The listing builds one solid part. Answer for the finished solid, in the listing's coordinates (mm). A direction names the side the tool comes from. Coordinates: 2 decimals unless noted, no trailing zeros. Order: outer loops, then holes, each group sorted by start corner. A loop starts at its lowest first (then second) coordinate and runs counter-clockwise, first axis right, second up. Notation, with made-up numbers: (-34, 6) -> (3, 6) arc R20 cw to (3, 21) -> close; hole circle Ø3 at (68.25, -1). An arc over 180 degrees is marked (long way). Write item = value, one per line.
from build123d import *

# Parameters (mm, degrees)
F0_W      = 96
F0_H      = 90
F1_DEPTH  = 18
F2_W      = 72
F2_H      = 38
F4_DEPTH  = 67
F6_DEPTH  = 38
F7_W      = 8
F7_H      = 12
F8_DEPTH  = 51.001
F10_DEPTH = 72.001
F11_W     = 20
F11_H     = 5
F12_DEPTH = 96
F13_W     = 46
F13_H     = 26
F14_DEPTH = 5
F16_DEPTH = 3
F17_W     = 3
F17_H     = 14
F18_DEPTH = 72
F19_R     = 2.99999


# Not quite as in the source:
# - a fillet or chamfer is up to 0.001 mm smaller than in the source, because OpenCascade refuses the exact size


with BuildPart() as f1:
    # F0 (on Top) → F1 (new body)
    with BuildSketch(Plane.XY):
        with Locations((48, 45)):
            Rectangle(F0_W, F0_H)
    extrude(amount=F1_DEPTH)

    # F2 (on face) → F4 (join, through all)
    with BuildSketch(Plane.XY.offset(18)):
        with Locations((48, 71)):
            Rectangle(F2_W, F2_H)
    extrude(amount=F4_DEPTH)

    # F5 (on face) → F6 (cut, through all)
    with BuildSketch(Plane.XZ.offset(-52)):
        Polygon((84, 52), (84, 85), (51, 85), align=None)
    extrude(amount=-F6_DEPTH, mode=Mode.SUBTRACT)

    # F7 (on face) → F8 (cut, through all)
    with BuildSketch(Plane(origin=(12, 0, 0), x_dir=(0, -1, 0), z_dir=(-1, 0, 0))):
        with Locations((-64, 79)):
            Rectangle(F7_W, F7_H)
    extrude(amount=-F8_DEPTH, mode=Mode.SUBTRACT)

    # F9 (on face) → F10 (cut, through all)
    with BuildSketch(Plane(origin=(12, 0, 0), x_dir=(0, -1, 0), z_dir=(-1, 0, 0))):
        Polygon((-90, 40), (-76, 85), (-90, 85), align=None)
    extrude(amount=-F10_DEPTH, mode=Mode.SUBTRACT)

    # F11 (on face) → F12 (cut, through all)
    with BuildSketch(Plane.YZ.offset(96)):
        with Locations((32, 2.5)):
            Rectangle(F11_W, F11_H)
    extrude(amount=-F12_DEPTH, mode=Mode.SUBTRACT)

    # F13 (on face) → F14 (join)
    with BuildSketch(Plane.XY.offset(18)):
        with Locations((48, 31.9999999999)):
            Rectangle(F13_W, F13_H)
        with BuildLine():
            Line((25, 18.9999999999), (25, 44.9999999999))
            ThreePointArc((25, 44.9999999999), (12, 31.9999999999), (25, 18.9999999999))
        make_face()
        with BuildLine():
            ThreePointArc((71, 18.9999999999), (84, 31.9999999999), (71, 44.9999999999))
            Line((71, 44.9999999999), (71, 18.9999999999))
        make_face()
    extrude(amount=F14_DEPTH)

    # F15 (on face) → F16 (cut)
    with BuildSketch(Plane.XY.offset(23)):
        with BuildLine():
            ThreePointArc((71, 25.9999999999), (77, 31.9999999999), (71, 37.9999999999))
            Line((71, 37.9999999999), (71, 25.9999999999))
        make_face()
        Polygon((25, 37.9999999999), (25, 31.9999999999), (25, 25.9999999999), (71, 25.9999999999), (71, 37.9999999999), align=None)
        with BuildLine():
            Line((25, 25.9999999999), (25, 31.9999999999))
            Line((25, 31.9999999999), (25, 37.9999999999))
            ThreePointArc((25, 37.9999999999), (19, 31.9999999999), (25, 25.9999999999))
        make_face()
    extrude(amount=-F16_DEPTH, mode=Mode.SUBTRACT)

    # F17 (on face) → F18 (cut, through all)
    with BuildSketch(Plane.YZ.offset(84)):
        with Locations((53.5, 25)):
            Rectangle(F17_W, F17_H)
    extrude(amount=-F18_DEPTH, mode=Mode.SUBTRACT)

    # F19 (radius 3 in the source; OpenCascade refuses exactly that, so slightly less here)
    f19_edges = [f1.edges().sort_by_distance(p)[0] for p in [
        (48, 55, 18),
        (48, 19, 18),
        (48, 55, 32),
        (96, 45, 18),
        (0, 45, 18),
        (96, 0, 9),
        (0, 0, 9),
    ]]
    fillet(f19_edges, radius=F19_R)


solid = f1.part
Q1. Section C-C, the plane z = 36.5 is taken. Give the vertices of the cut face in (x, y).
The answers:
outline = (12, 52) -> (84, 52) -> (84, 90) -> (12, 90) -> close
Q2. Section B-B, the plane y = 64 is taken. Give the vertices of the cut face in (x, z).
The answers:
outline = (0, 0) -> (96, 0) -> (96, 15) arc R3 ccw to (93, 18) -> (84, 18) -> (84, 52) -> (63, 73) -> (12, 73) -> (12, 18) -> (3, 18) arc R3 ccw to (0, 15) -> close
Q3. A tool of negligible diameter and unlimited length cuts with its end or side. For faces 4 (the face through (37, 64, 73)), 5 (the face through (47, 52, 58)), 6 (the face through (84, 32, 22)), 7 (the face through (49, 22, 2)), 8 (the face through (48, 26, 22)), from which of +Z, -Z, +X, -X, +Y, -Y can it reach the whole face along a straight path? Write none if from no direction.
The answers:
face_4 = +Z, +X, -X
face_5 = +Z, +X, -X, -Y
face_6 = +Z, +X
face_7 = -Z, +X, -X
face_8 = +Z
Q4. The mould has two halves that part along Z. Classify faces 1 (the face through (0, 46, 7)), 2 (the face through (47.5, 54.1, 18.86)), 3 (the face through (47.4, 15.6, 18)): released by +Z, released by -Z, zero draft, split by the parting line, or undercut.
The answers:
face_1 = zero draft
face_2 = undercut
face_3 = released by +Z
Q5. Each of these flat-tipped pins is pushed along its axis until it touches: pin 1 Ø4 at (x, y) = (23, 76) entering from -Z; pin 2 Ø19 at (y, z) = (79, 53.5) entering from -X; pin 3 Ø4 at (x, y) = (28, 65) entering from +Z; pin 4 Ø8 at (x, y) = (42.5, 31.5) entering from -Z. Where does it stop, or does it pass through?
The answers:
pin_1 = 0
pin_2 = 12
pin_3 = 73
pin_4 = 5
Q6. Find the intervals of material crossed by line 1 along Z through (x, y) = (14, 45.5); line 2 along Z through (x, y) = (25, 62.5); line 3 along Y through (x, z) = (32.5, 72), in increasing order.
The answers:
line_1 = 0 to 18
line_2 = 0 to 73
line_3 = 52 to 80.04
